Can you work these out from the model? Positions are in its coordinate system, mm. A direction names the side the tool comes from. Coordinates: 2 decimals unless noted, no trailing zeros. Order: outer loops, then holes, each group sorted by start corner. A loop starts at its lowest first (then second) coordinate and runs counter-clockwise, first axis right, second up. Notation, with made-up numbers: (25, -2) -> (50, -2) arc R21 ccw to (50, 13) -> close; hole circle Ø5 at (60, 58). An arc over 180 degrees is marked (long way). Return JSON: item names as keys, results as strings. Group by question number.
1) If we section it at C-C, the plane x = 0: Please give me the cut outline in (y, z), then the cut area to 3 significant figures.
2) If we section it at B-B, the plane z = 0: Please give me the cut outline in (x, y), then the cut area to 3 significant figures.
3) If I drill on probe 1 along Z at (x, y) = (0.25, 17); probe 2 along Y at (x, z) = (-5.25, 1.75); probe 3 along Y at (x, z) = (7.75, 3.25), over which ranges is the centre line in solid material (lowest first)? Write a range as from..to.
4) If we section it at A-A, the plane y = 13.5: Please give me the cut outline in (x, z), then the cut area to 3 significant figures.
5) If we section it at D-D, the plane y = 18: Please give me the cut outline in (x, z).
6) Thinking about a two-plate mould opening in X: for faces 4 (the flat face through (5.406, 12.535, -6.766)), 5 (the flat face through (0, 0, 0)), 6 (the flat face through (-3.157, 12.535, -8.065)), which applies, +X half, -X half, draft (parallel to the pull), parting line (faces both ways), or undercut?
7) For faces 1 (the flat face through (-8.563, 12.535, -1.299)), 2 (the flat face through (-2, 15, 5)), 3 (the flat face through (6, 10, -4)), which set-ups out of +Z, -Z, +X, -X, +Y, -Y let a thin tool reach every point of the face, with its end or its side?
8) For pin 1 (6 mm diameter, centred on y = 6.5, z = -4, fed in from -X); pin 2 (2 mm diameter, centred on y = 19, z = -1.5, fed in from +X); pin 3 (6 mm diameter, centred on x = 4, y = 14.5, fed in from +Z), each with a flat end and sliding along its axis, tell me the tip position at first contact or that it passes through.
from build123d import *

# Parameters (mm, degrees)
SKETCH_2_OUTSIDE_W  = 29.55
SKETCH_2_OUTSIDE_H  = 29.55
CUT_EXTRUDE_1_DEPTH = 16


with BuildPart() as part:
    # Эскиз1 → Повернуть1 (revolve)
    with BuildSketch(Plane.XY):
        Polygon((0, 0), (7, 0), (7, 10), (10, 10), (10, 15), (5, 15), (5, 21.744186047), (1.744186047, 25), (0, 25), align=None)
    revolve(axis=Axis((0, 25, 0), (0, -1, 0)))

    # Эскиз2 outside → Вырез-Вытянуть1 (cut, through all)
    with BuildSketch(Plane(origin=(0, 15, 0), x_dir=(1, 0, 0), z_dir=(0, 1, 0))):
        Rectangle(SKETCH_2_OUTSIDE_W, SKETCH_2_OUTSIDE_H)
        Polygon((7.862707781, -6.178820789), (9.282369659, 3.719894287), (1.419661878, 9.898715076), (-7.862707781, 6.178820789), (-9.282369659, -3.719894287), (-1.419661878, -9.898715076), align=None, mode=Mode.SUBTRACT)
    extrude(amount=-CUT_EXTRUDE_1_DEPTH, mode=Mode.SUBTRACT)


solid = part.part
Result sheet:
{
 "1": {"outline": "(0, -7) -> (10, -7) -> (10, -9.33) -> (15, -9.33) -> (15, -5) -> (21.74, -5) -> (25, -1.74) -> (25, 1.74) -> (21.74, 5) -> (15, 5) -> (15, 9.33) -> (10, 9.33) -> (10, 7) -> (0, 7) -> close", "area": "323 mm2"},
 "2": {"outline": "(-8.75, 10) -> (-7, 10) -> (-7, 0) -> (7, 0) -> (7, 10) -> (8.75, 10) -> (8.75, 15) -> (5, 15) -> (5, 21.74) -> (1.74, 25) -> (-1.74, 25) -> (-5, 21.74) -> (-5, 15) -> (-8.75, 15) -> close", "area": "317 mm2"},
 "3": {"probe 1": "z = -4.99..4.99", "probe 2": "y = 0..15", "probe 3": "y = 10..15"},
 "4": {"outline": "(-9.28, 3.72) -> (-7.86, -6.18) -> (1.42, -9.9) -> (9.28, -3.72) -> (7.86, 6.18) -> (-1.42, 9.9) -> close", "area": "260 mm2"},
 "5": {"outline": "circle Ø10 at (0, 0)"},
 "6": {"face 4": "+X half", "face 5": "draft", "face 6": "-X half"},
 "7": {"face 1": "-Z, -X, +Y, -Y", "face 2": "+Y", "face 3": "-Y"},
 "8": {"pin 1": "stops at x = -6.93", "pin 2": "stops at x = 4.97", "pin 3": "stops at z = 8.93"}
}
